from build123d import *

# Parameters (mm, degrees)
SKETCH1_W           = 74
SKETCH1_H           = 24
SKETCH1_W_2         = 68
SKETCH1_H_2         = 18
BOSS_EXTRUDE1_DEPTH = 20
SKETCH1_3_W         = 74
SKETCH1_3_H         = 24
SKETCH1_3_W_2       = 68
SKETCH1_3_H_2       = 18
BOSS_EXTRUDE2_DEPTH = 3
CUT_EXTRUDE1_REACH  = 61.463
SKETCH4_W           = 18
SKETCH4_H           = 10


with BuildPart() as part:
    # Sketch1 → Boss-Extrude1 (new body)
    with BuildSketch(Plane(origin=(0, 0, 0), x_dir=(1, 0, 0), z_dir=(0, 1, 0))):
        with Locations((14.912280702, -12.336842105)):
            Rectangle(SKETCH1_W, SKETCH1_H)
        with Locations((14.912280702, -12.336842105)):
            Rectangle(SKETCH1_W_2, SKETCH1_H_2, mode=Mode.SUBTRACT)
    extrude(amount=BOSS_EXTRUDE1_DEPTH)

    # Sketch1_3 → Boss-Extrude2 (add)
    # profile 1 of 2: a face of its own
    with BuildSketch(Plane(origin=(0, 0, 0), x_dir=(1, 0, 0), z_dir=(0, 1, 0))):
        with Locations((14.912280702, -12.336842105)):
            Rectangle(SKETCH1_3_W, SKETCH1_3_H)
        with Locations((14.912280702, -12.336842105)):
            Rectangle(SKETCH1_3_W_2, SKETCH1_3_H_2, mode=Mode.SUBTRACT)
    # profile 2 of 2: a face of its own
    with BuildSketch(Plane(origin=(0, 0, 0), x_dir=(1, 0, 0), z_dir=(0, 1, 0))):
        with Locations((14.912280702, -12.336842105)):
            Rectangle(SKETCH1_3_W_2, SKETCH1_3_H_2)
    extrude(amount=-BOSS_EXTRUDE2_DEPTH)

    # Sketch4 → Cut-Extrude1 (cut, up to next)
    with BuildSketch(Plane(origin=(0, 0, 21.336842105), x_dir=(-1, 0, 0), z_dir=(0, 0, -1)), mode=Mode.PRIVATE) as cut_extrude1_sk1:
        with Locations((-14.912280702, 15)):
            Rectangle(SKETCH4_W, SKETCH4_H)
    cut_extrude1_tool1 = extrude(cut_extrude1_sk1.sketch, amount=-CUT_EXTRUDE1_REACH, mode=Mode.PRIVATE) & part.part
    add(cut_extrude1_tool1.solids().sort_by_distance((14.912281, 15, 21.336842))[0], mode=Mode.SUBTRACT)


solid = part.part
Design review of the part built by this model. Coordinates are the model's own, in mm. A direction names the side the tool comes from. Round coordinates to 2 decimals unless told otherwise and drop trailing zeros. Write each loop counter-clockwise with the first axis right and the second up, starting at its lowest first coordinate (ties: lowest second). Pieces come first, ordered by that corner, then holes.
Item 1: Wall thickness on L1, parallel to Z at x = 38, y = 8.5; L2, parallel to X at y = 19.25, z = 17; L3, parallel to X at y = 13.25, z = 21.75: over which ranges is each line inside the solid? List them lowest first.
Item 2: For pin 1 Ø0.9 at (x, z) = (19, 23) entering from +Y; pin 2 Ø6 at (x, z) = (11.5, 14) entering from +Y, all flat-tipped, find the tip position at first contact; note any pin that passes through.
Item 3: Consider section C-C on x = 17. Give the boundary of the cut face in (y, z).
Item 4: For faces 1 (the flat face through (12, 20, 3)), 2 (the flat face through (5.912, 15, 23)), 3 (the flat face through (48.912, 10, 12)), list the 3-axis set-ups (+Z, -Z, +X, -X, +Y, -Y) from which the entire face can be reached by the end or side of a thin tool; tool diameter is ignored.
Item 5: Consider section A-A on y = 8. Give the boundary of the cut face in (x, z), and give its area (3 significant figures).
Item 6: Consider section B-B on z = 16.5. Give the boundary of the cut face in (x, y), and give its area (3 significant figures).
Item 7: Consider section D-D on y = 17.5. Give the boundary of the cut face in (x, z).
Item 8: Draft analysis for pull direction Z (two halves, no side actions). For faces 4 (the flat face through (14, 9, 0.337)), 5 (the flat face through (14, 9, 24.337)), 6 (the flat face through (15, 10, 23)), 7 (the flat face through (14, 0, 12)), state which applies: released by +Z, released by -Z, zero draft, split by the parting line, or undercut.
Check values:
1. L1: z = 0.34 to 3.34, 21.34 to 24.34
1. L2: x = -22.09 to -19.09, 48.91 to 51.91
1. L3: x = -22.09 to 5.91, 23.91 to 51.91
2. pin 1: stops at y = 10
2. pin 2: stops at y = 0
3. outline: (-3, 0.34) - (20, 0.34) - (20, 3.34) - (0, 3.34) - (0, 21.34) - (10, 21.34) - (10, 24.34) - (-3, 24.34) - close
4. face 1: +Z, -Z, +X, -X, +Y
4. face 2: +Z, +Y
4. face 3: +Y
5. outline: (-22.09, 0.34) - (51.91, 0.34) - (51.91, 24.34) - (-22.09, 24.34) - close; hole (-19.09, 3.34) - (48.91, 3.34) - (48.91, 21.34) - (-19.09, 21.34) - close
5. area: 552 mm2
6. outline: (-22.09, -3) - (51.91, -3) - (51.91, 20) - (48.91, 20) - (48.91, 0) - (-19.09, 0) - (-19.09, 20) - (-22.09, 20) - close
6. area: 342 mm2
7. outline: (-22.09, 0.34) - (51.91, 0.34) - (51.91, 24.34) - (23.91, 24.34) - (23.91, 21.34) - (48.91, 21.34) - (48.91, 3.34) - (-19.09, 3.34) - (-19.09, 21.34) - (5.91, 21.34) - (5.91, 24.34) - (-22.09, 24.34) - close
8. face 4: released by -Z
8. face 5: released by +Z
8. face 6: zero draft
8. face 7: undercut
